Study the drawing (mm; zero at the part's minimum x, y, z) and answer. A direction names the side the tool comes from. Give positions to 0.01 mm unless a question says otherwise; leave off trailing zeros. Loops run counter-clockwise (first coordinate to the right, second up) from the corner with the lowest first, then second, coordinate; pieces in that order, holes last. Notation, with made-up numbers: (22.25, 7.25) - (71.25, 7.25) arc R29 ccw to (71.25, 35.25) - close; hole circle Ø9 at (13.25, -18). An arc over 180 degrees is marked (long way). Write item = value, one per line. Start each with the question number.
1) Consider probe 1 along X at (y, z) = (52, 17.5); probe 2 along Y at (x, z) = (45, 5.75); probe 3 along X at (y, z) = (170, 1.75). Determine where each line is inside the solid, lowest interval first.
2) Which of the six approach directions +Z, -Z, +X, -X, +Y, -Y give full straight-line access (tool end or side, diameter ignored) to the marked faces 1 and 2?
3) The part is cut by section D-D on y = 141. Write down the section's boundary in (x, z).
4) The mould has two halves that part along X. Classify the marked faces 3, 4 and 5: +X half, -X half, draft (parallel to the pull), parting line (faces both ways), or undercut.
5) The part is cut by section B-B on z = 4. Write down the section's boundary in (x, y).
6) The part is cut by section C-C on x = 71.5. Write down the section's boundary in (y, z).
7) Flat-ended cylindrical pins translate along their axes: P1, Ø10, axis at x = 51.5, z = 14.5, coming from the -Y side; P2, Ø6, axis at x = 56, z = 16.5, coming from the +Y side; P3, Ø0.5, axis at x = 1, z = 7, coming from the +Y side; P4, Ø3.5, axis at y = 167.63, z = 9.53, coming from the -X side. Find the tip coordinate at first contact, or state that the pin passes through.
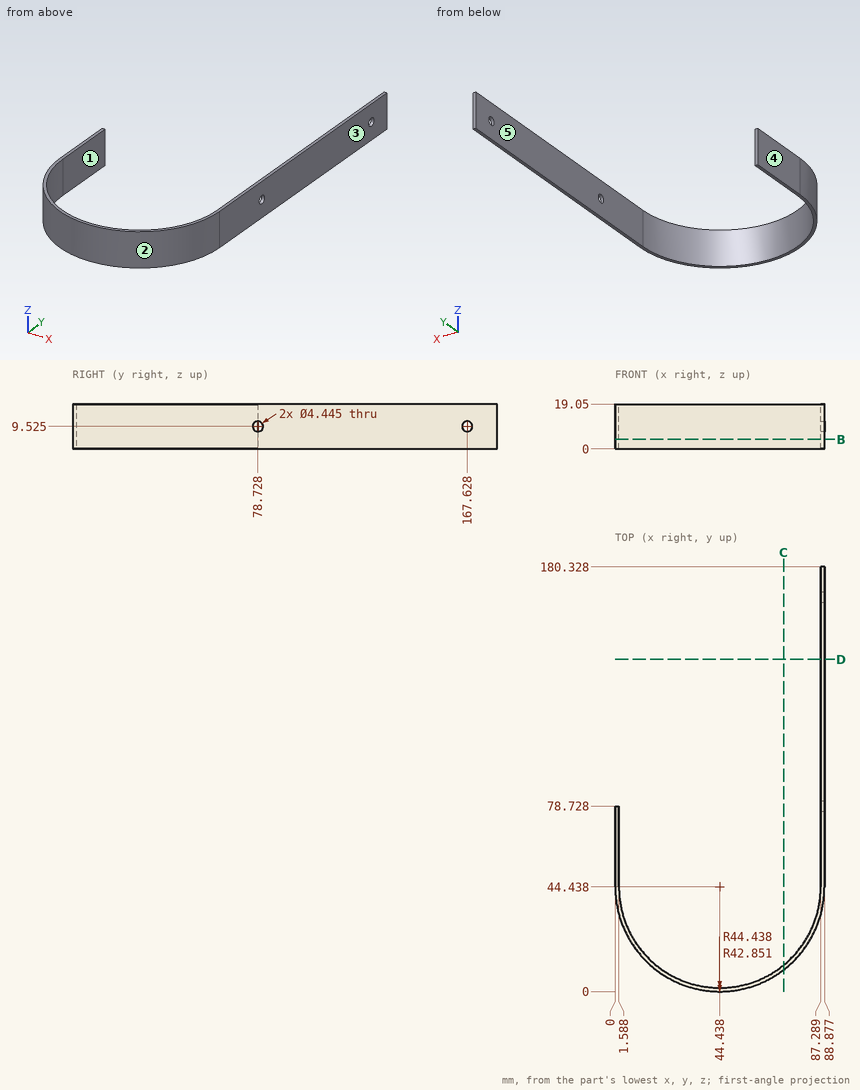
Answer below:
q1.probe_1 = 0 to 1.59, 87.29 to 88.88
q1.probe_2 = 0 to 1.59
q1.probe_3 = 87.29 to 88.88
q2.face_1 = +Z, -Z, +Y
q2.face_2 = +Z, -Z, -Y
q3.outline = (87.29, 0) - (88.88, 0) - (88.88, 19.05) - (87.29, 19.05) - close
q4.face_3 = +X half
q4.face_4 = -X half
q4.face_5 = undercut
q5.outline = (0, 44.44) arc R44.44 ccw to (88.88, 44.44) - (88.88, 180.33) - (87.29, 180.33) - (87.29, 44.44) arc R42.85 cw to (1.59, 44.44) - (1.59, 78.73) - (0, 78.73) - close
q6.outline = (9.19, 0) - (11.21, 0) - (11.21, 19.05) - (9.19, 19.05) - close
q7.P1 = 0.05
q7.P2 = 4.14
q7.P3 = 78.73
q7.P4 = through
